For this review, take the finished solid that the model builds, in its own axes (mm). A direction names the side the tool comes from. Round coordinates to 2 decimals unless told otherwise and drop trailing zeros. Write each loop counter-clockwise with the first axis right and the second up, starting at its lowest first coordinate (ties: lowest second). Pieces come first, ordered by that corner, then holes. Notation, with made-up numbers: M -38,52.5 L 3,52.5 A21 cw 3,58.5 Z; hole C 21,-26 d9. An arc over 180 degrees is marked long. Answer in a Markdown table with one row per item.
```python
from build123d import *

# Parameters (mm, degrees)
BOX003_W     = 10
BOX003_H     = 5
BOX003_DEPTH = 2
BOX001_W     = 10
BOX001_H     = 10
BOX001_DEPTH = 20
BOX002_W     = 12
BOX002_H     = 23
BOX002_DEPTH = 4
BOX_W        = 36.5
BOX_H        = 33
BOX_DEPTH    = 4


with BuildPart() as box003:
    # Box003 → Box003 (new body)
    with BuildSketch(Plane(origin=(26.5, 14, 18.5), x_dir=(1, 0, 0), z_dir=(0, 0, 1))):
        with Locations((5, 2.5)):
            Rectangle(BOX003_W, BOX003_H)
    extrude(amount=BOX003_DEPTH)


with BuildPart() as cut001:
    # Box001 → Box001 (new body)
    with BuildSketch(Plane(origin=(26.5, 11.5, 4), x_dir=(1, 0, 0), z_dir=(0, 0, 1))):
        with Locations((5, 5)):
            Rectangle(BOX001_W, BOX001_H)
    extrude(amount=BOX001_DEPTH)

    # Cut001: cut Box003
    add(box003.part, mode=Mode.SUBTRACT)


with BuildPart() as box002:
    # Box002 → Box002 (new body)
    with BuildSketch(Plane(origin=(0, 5, 0), x_dir=(1, 0, 0), z_dir=(0, 0, 1))):
        with Locations((6, 11.5)):
            Rectangle(BOX002_W, BOX002_H)
    extrude(amount=BOX002_DEPTH)


with BuildPart() as fusion:
    # Box → Box (new body)
    with BuildSketch(Plane.XY):
        with Locations((18.25, 16.5)):
            Rectangle(BOX_W, BOX_H)
    extrude(amount=BOX_DEPTH)

    # Cut: cut Box002
    add(box002.part, mode=Mode.SUBTRACT)

    # Fusion: union Cut001
    add(cut001.part)


solid = fusion.part
```
Q1. For probe 1 along Y at (x, z) = (3, 2.25); probe 2 along Y at (x, z) = (27.5, 15.75); probe 3 along Z at (x, y) = (29, 3.5), list the stretches that pass through material, from the lowest coordinate up.
Found:
| item | result |
|---|---|
| probe 1 | 0 to 5, 28 to 33 |
| probe 2 | 11.5 to 21.5 |
| probe 3 | 0 to 4 |
Q2. Take a section at C-C (y = 30). State the section outline as (x, z) points, then the cut area to 3 significant figures.
Found:
| item | result |
|---|---|
| outline | M 0,0 L 36.5,0 L 36.5,4 L 0,4 Z |
| area | 146 mm² |
Q3. Machinability: for faces 4 (the face through (31, 14, 19)), 5 (the face through (6, 5, 2)), 6 (the face through (31, 21.5, 14)), 7 (the face through (0, 30, 2)), 8 (the face through (26.5, 16, 14)), which of the approach directions +Z, -Z, +X, -X, +Y, -Y give a long, thin tool a straight path to every point of the face, cutting with its end or side? Answer none if there is none.
Found:
| item | result |
|---|---|
| face 4 | +X, -X |
| face 5 | +Z, -Z, -X |
| face 6 | +Z, +X, -X, +Y |
| face 7 | +Z, -Z, -X, +Y, -Y |
| face 8 | +Z, -X, +Y, -Y |
Q4. Take a section at A-A (x = 11). State the section outline as (y, z) points.
Found:
| item | result |
|---|---|
| outline | M 0,0 L 5,0 L 5,4 L 0,4 Z; M 28,0 L 33,0 L 33,4 L 28,4 Z |
Q5. Take a section at D-D (x = 17.5). State the section outline as (y, z) points.
Found:
| item | result |
|---|---|
| outline | M 0,0 L 33,0 L 33,4 L 0,4 Z |
Q6. Insertion check: P1, Ø3, axis at x = 31, z = 15.5, coming from the +Y side; P2, Ø5, axis at y = 16.5, z = 10.5, coming from the -X side; P3, Ø5, axis at x = 13, y = 13, coming from the +Z side. Each pin has a flat end and moves straight along its axis. Give the tip position at first contact, or say it passes through.
Found:
| item | result |
|---|---|
| P1 | y = 21.5 |
| P2 | x = 26.5 |
| P3 | z = 4 |
Q7. Mouldability with a two-part tool opening along Z and no side actions: class faces 1 (the face through (31, 17, 20.5)), 2 (the face through (31, 11.5, 14)), 3 (the face through (31, 17, 24)) as +Z half, -Z half, draft (parallel to the pull), parting line (faces both ways), or undercut.
Found:
| item | result |
|---|---|
| face 1 | undercut |
| face 2 | draft |
| face 3 | +Z half |
Q8. Take a section at B-B (z = 3). State the section outline as (x, y) points.
Found:
| item | result |
|---|---|
| outline | M 0,0 L 36.5,0 L 36.5,33 L 0,33 L 0,28 L 12,28 L 12,5 L 0,5 Z |
